from build123d import *

# Parameters (mm, degrees)
F1_DEPTH      = 140
F3_DEPTH      = 3
F3_DEPTH_BACK = 3
F5_DEPTH      = 3
F5_DEPTH_BACK = 3


with BuildPart() as f1:
    # F0 (on Top) → F1 (new body)
    with BuildSketch(Plane.XY):
        Polygon((-9, 0), (0, 0), (9, 0), (9, -3.2), (6, -3.2), (6, -5.7), (12, -5.7), (12, 4), (6.25, 4), (6.25, 7.5), (9, 7.5), (9, 10.6), (3.5, 10.6), (3.5, 9.1), (0, 9.1), (-3.5, 9.1), (-3.5, 10.6), (-9, 10.6), (-9, 7.5), (-6.25, 7.5), (-6.25, 4), (-12, 4), (-12, -5.7), (-6, -5.7), (-6, -3.2), (-9, -3.2), align=None)
    extrude(amount=F1_DEPTH)

    # F2 (on Right) → F3 (join, two sides)
    with BuildSketch(Plane.YZ) as f3_sk:
        Polygon((0, 52.5), (-3.5, 51), (-3.5, 49), (0, 47.5), align=None)
    extrude(amount=F3_DEPTH)
    extrude(f3_sk.sketch, amount=-F3_DEPTH_BACK)

    # F4 (on Right) → F5 (join, two sides)
    with BuildSketch(Plane.YZ) as f5_sk:
        Polygon((7.5, 128), (7.5, 114), (10.5, 119), (9, 120), (9, 122), (10.5, 123), align=None)
    extrude(amount=F5_DEPTH)
    extrude(f5_sk.sketch, amount=-F5_DEPTH_BACK)


solid = f1.part
Geometry check sheet. Reference: the model listing, model coordinates, mm. A direction names the side the tool comes from. Round coordinates to 2 decimals unless told otherwise and drop trailing zeros. Loops run counter-clockwise (first coordinate to the right, second up) from the corner with the lowest first, then second, coordinate; pieces in that order, holes last. Notation, with made-up numbers: (-32, -39.75) - (8, -39.75) arc R10 cw to (8, -29.75) - close; hole circle Ø2 at (-10.5, -1.75). An arc over 180 degrees is marked (long way). Answer as CSV lines item,"result".
(1) Release check for a two-part mould opening along X. For faces 5 (the face through (12, -1, 69)), 6 (the face through (8, 7.5, 69)), 7 (the face through (3, -1, 50)) record: released by +X, released by -X, zero draft, split by the parting line, or undercut.
Output values:
face 5,"released by +X"
face 6,"zero draft"
face 7,"undercut"
(2) Cross-section at B-B, the plane x = 1.25. Enter the section's corners in (y, z).
Output values:
outline,"(-3.5, 49) - (0, 47.5) - (0, 0) - (9.1, 0) - (9.1, 116.67) - (10.5, 119) - (9.1, 119.93) - (9.1, 122.07) - (10.5, 123) - (9.1, 125.33) - (9.1, 140) - (0, 140) - (0, 52.5) - (-3.5, 51) - close"
(3) Cross-section at C-C, the plane y = 5.25. Enter the section's corners in (x, z), and give its area (3 significant figures).
Output values:
outline,"(-6.25, 0) - (6.25, 0) - (6.25, 140) - (-6.25, 140) - close"
area,"1,750 mm²"
(4) Depth check by flat-ended pin: pin 1 Ø4 at (x, z) = (0, 40.5) entering from -Y; pin 2 Ø3 at (y, z) = (7.5, 16) entering from +X; pin 3 Ø0.9 at (y, z) = (9.5, 103.5) entering from -X. Enter the tip coordinate at first touch or a pass-through.
Output values:
pin 1,"stops at y = 0"
pin 2,"stops at x = 9"
pin 3,"stops at x = -9"
(5) Cross-section at A-A, the plane z = 22.5. Enter the section's corners in (x, y), and give its area (3 significant figures).
Output values:
outline,"(-12, -5.7) - (-6, -5.7) - (-6, -3.2) - (-9, -3.2) - (-9, 0) - (9, 0) - (9, -3.2) - (6, -3.2) - (6, -5.7) - (12, -5.7) - (12, 4) - (6.25, 4) - (6.25, 7.5) - (9, 7.5) - (9, 10.6) - (3.5, 10.6) - (3.5, 9.1) - (-3.5, 9.1) - (-3.5, 10.6) - (-9, 10.6) - (-9, 7.5) - (-6.25, 7.5) - (-6.25, 4) - (-12, 4) - close"
area,"234 mm²"
(6) Material ranges on line 1 along Y through (x, z) = (-8.5, 54.5); line 2 along X through (y, z) = (-4.25, 90); line 3 along X through (y, z) = (-1.5, 110.5), recorded low to high.
Output values:
line 1,"y = -5.7 to -3.2, 0 to 4, 7.5 to 10.6"
line 2,"x = -12 to -6, 6 to 12"
line 3,"x = -12 to -9, 9 to 12"
(7) Set-up check for faces 1 (the face through (-6, -4, 69)), 2 (the face through (0.04, 9.81, 124.15)), 3 (the face through (-9, -2, 69)), 4 (the face through (-0.04, -1.77, 48.26)): record each of +Z, -Z, +X, -X, +Y, -Y from which the full face is reachable in a straight line by a thin tool's end or side.
Output values:
face 1,"+Z, -Z, -Y"
face 2,"+Z, +Y"
face 3,"+Z, -Z"
face 4,"-Z, -Y"
